The model under review builds one solid part; all positions refer to its coordinate system, in mm. Give positions to 0.01 mm unless a question says otherwise; leave off trailing zeros. Loops run counter-clockwise (first coordinate to the right, second up) from the corner with the lowest first, then second, coordinate; pieces in that order, holes last. Notation, with made-up numbers: (70.5, -3.75) - (120.5, -3.75) arc R8 ccw to (120.5, 0.25) - close; hole circle Ø3 at (33, -9). An arc over 180 degrees is marked (long way). Answer as a JSON object with one key per item and string values.
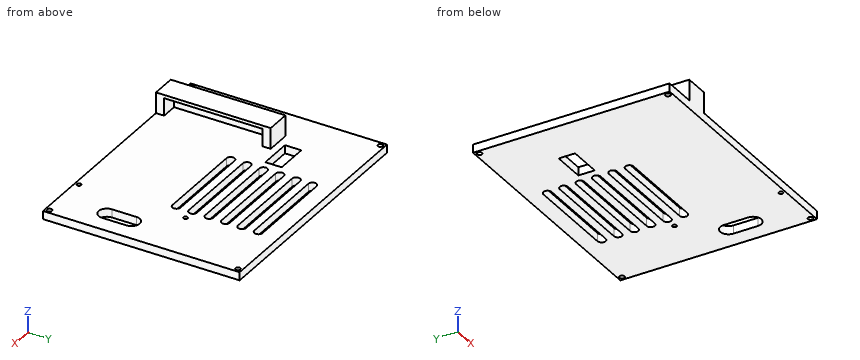
Autodesk Fusion 360 part; units mm, degrees
sketch "スケッチ1" plane through (0, 0, 0) normal (0, 0, 1) x (1, 0, 0)
  line L0 (75, -45) -> (-75, -45)
  line L1 (-75, -45) -> (-75, 75)
  line L2 (-75, 75) -> (75, 75)
  line L3 (75, 75) -> (75, -45)
  line L4 (-115.7726, 0) -> (130, 0)
  dimension "d1" = 150
  dimension "d41" = 75
  dimension "d42" = 45
extrude "押し出し1" add sketch "スケッチ1" along normal blind 5
sketch "スケッチ2" plane through (0, 0, 5) normal (0, 0, 1) x (-1, 0, 0)
  line L0 (-75, -75) -> (75, -75)
  line L1 (75, -75) -> (75, 45)
  line L2 (75, 45) -> (-75, 45)
  line L3 (-75, 45) -> (-75, -75)
  circle A0 centre (72.5, -72.5) radius 1.5
  line L4 (0, -100) -> (0, -20)
  circle A1 centre (-72.5, -72.5) radius 1.5
  line L5 (50, 0) -> (-80, 0)
  circle A2 centre (72.5, 72.5) radius 1.5
  circle A3 centre (-72.5, 72.5) radius 1.5
  dimension "d5" = 3
  dimension "d6" = 2.5
  dimension "d7" = 2.5
extrude "押し出し2" cut sketch "スケッチ2" against normal blind 5 contours A0 | A1 | A2 | A3
sketch "スケッチ3" plane through (0, 0, 5) normal (0, 0, 1) x (-1, 0, 0)
  circle A0 centre (-72.5, -72.5) radius 1.5
  circle A1 centre (72.5, -72.5) radius 1.5
  line L0 (-75, -75) -> (75, -75)
  line L1 (75, -75) -> (75, 45)
  line L2 (75, 45) -> (-75, 45)
  line L3 (-75, 45) -> (-75, -75)
  line L4 (47, -39.5) -> (27, -39.5)
  line L5 (27, -39.5) -> (27, -29.5)
  line L6 (27, -29.5) -> (47, -29.5)
  line L7 (47, -29.5) -> (47, -39.5)
  dimension "d10" = 28
  dimension "d11" = 45.5
  dimension "d12" = 10
  dimension "d13" = 20
extrude "押し出し3" cut sketch "スケッチ3" against normal blind 5 contours L4 L5 L6 L7
sketch "スケッチ4" plane through (0, 0, 5) normal (0, 0, 1) x (-1, 0, 0)
  line L0 (27, -39.5) -> (27, -29.5)
  line L1 (27, -29.5) -> (47, -29.5)
  line L2 (47, -29.5) -> (47, -39.5)
  line L3 (47, -39.5) -> (27, -39.5)
  circle A0 centre (-72.5, -72.5) radius 1.5
  circle A1 centre (72.5, -72.5) radius 1.5
  line L4 (-75, -75) -> (75, -75)
  line L5 (75, -75) -> (75, 45)
  line L6 (75, 45) -> (-75, 45)
  line L7 (-75, 45) -> (-75, -75)
  line L8 (20, -65) -> (-35, -65)
  line L9 (-35, -60) -> (20, -60)
  line L10 (20, -55) -> (-35, -55)
  line L11 (-35, -50) -> (20, -50)
  line L12 (20, -45) -> (-35, -45)
  line L13 (-35, -40) -> (20, -40)
  line L14 (20, -35) -> (-35, -35)
  line L15 (-35, -30) -> (20, -30)
  line L16 (20, -25) -> (-35, -25)
  line L17 (-35, -20) -> (20, -20)
  line L18 (20, -15) -> (-35, -15)
  line L19 (-35, -10) -> (20, -10)
  arc A2 (20, -65) -> (20, -60) centre (20, -62.5) ccw
  arc A3 (20, -55) -> (20, -50) centre (20, -52.5) ccw
  arc A4 (20, -45) -> (20, -40) centre (20, -42.5) ccw
  arc A5 (20, -35) -> (20, -30) centre (20, -32.5) ccw
  arc A6 (20, -25) -> (20, -20) centre (20, -22.5) ccw
  arc A7 (20, -15) -> (20, -10) centre (20, -12.5) ccw
  arc A8 (-35, -10) -> (-35, -15) centre (-35, -12.5) ccw
  arc A9 (-35, -20) -> (-35, -25) centre (-35, -22.5) ccw
  arc A10 (-35, -30) -> (-35, -35) centre (-35, -32.5) ccw
  arc A11 (-35, -40) -> (-35, -45) centre (-35, -42.5) ccw
  arc A12 (-35, -50) -> (-35, -55) centre (-35, -52.5) ccw
  arc A13 (-35, -60) -> (-35, -65) centre (-35, -62.5) ccw
extrude "押し出し4" cut sketch "スケッチ4" against normal blind 5 contours L8 L9 A2 A13 | L10 L11 A3 A12 | L12 L13 A4 A11 | L14 L15 A5 A10 | L16 L17 A6 A9 | L18 L19 A7 A8
sketch "スケッチ5" plane through (0, 0, 5) normal (0, 0, 1) x (-1, 0, 0)
  line L0 (-35, -30) -> (20, -30)
  arc A0 (20, -35) -> (20, -30) centre (20, -32.5) ccw
  line L1 (20, -35) -> (-35, -35)
  arc A1 (-35, -30) -> (-35, -35) centre (-35, -32.5) ccw
  line L2 (-35, -60) -> (20, -60)
  arc A2 (20, -65) -> (20, -60) centre (20, -62.5) ccw
  line L3 (20, -65) -> (-35, -65)
  arc A3 (-35, -60) -> (-35, -65) centre (-35, -62.5) ccw
  line L4 (-35, -50) -> (20, -50)
  arc A4 (20, -55) -> (20, -50) centre (20, -52.5) ccw
  line L5 (20, -55) -> (-35, -55)
  arc A5 (-35, -50) -> (-35, -55) centre (-35, -52.5) ccw
  line L6 (-35, -20) -> (20, -20)
  arc A6 (20, -25) -> (20, -20) centre (20, -22.5) ccw
  line L7 (20, -25) -> (-35, -25)
  arc A7 (-35, -20) -> (-35, -25) centre (-35, -22.5) ccw
  line L8 (-35, -10) -> (20, -10)
  arc A8 (20, -15) -> (20, -10) centre (20, -12.5) ccw
  line L9 (20, -15) -> (-35, -15)
  arc A9 (-35, -10) -> (-35, -15) centre (-35, -12.5) ccw
  line L10 (-35, -40) -> (20, -40)
  arc A10 (20, -45) -> (20, -40) centre (20, -42.5) ccw
  line L11 (20, -45) -> (-35, -45)
  arc A11 (-35, -40) -> (-35, -45) centre (-35, -42.5) ccw
  line L12 (27, -39.5) -> (27, -29.5)
  line L13 (27, -29.5) -> (47, -29.5)
  line L14 (47, -29.5) -> (47, -39.5)
  line L15 (47, -39.5) -> (27, -39.5)
  circle A12 centre (-72.5, -72.5) radius 1.5
  circle A13 centre (72.5, -72.5) radius 1.5
  line L16 (-75, -75) -> (75, -75)
  line L17 (75, -75) -> (75, 45)
  line L18 (75, 45) -> (-75, 45)
  line L19 (-75, 45) -> (-75, -75)
  line L20 (50, -20) -> (40, -20)
  line L21 (40, 40) -> (50, 40)
  line L22 (50, 40) -> (50, -20)
  line L23 (55, -25) -> (40, -25)
  line L24 (40, 45) -> (55, 45)
  line L25 (55, 45) -> (55, -25)
  line L26 (40, -25) -> (40, -20)
  line L27 (40, 40) -> (40, 45)
  circle A14 centre (-52.5, -22.5) radius 1.5
  circle A15 centre (-52.5, 42.5) radius 1.5
  dimension "d18" = 60
  dimension "d20" = 3
  dimension "d21" = 3
  dimension "d22" = 2.5
  dimension "d25" = 2.5
extrude "押し出し5" add sketch "スケッチ5" along normal blind 10.7 contours L18 L20 L21 L22 L23 L24 L25 L26 L27
sketch "スケッチ7" plane through (0, 0, 15.7) normal (0, 0, 1) x (-1, 0, 0)
  line L0 (50, 40) -> (50, -20)
  line L1 (50, -20) -> (40, -20)
  line L2 (40, -20) -> (40, -25)
  line L3 (40, -25) -> (55, -25)
  line L4 (55, -25) -> (55, 45)
  line L5 (55, 45) -> (40, 45)
  line L6 (40, 45) -> (40, 40)
  line L7 (40, 40) -> (50, 40)
  line L8 (55, -25) -> (40, -25)
  line L9 (40, -25) -> (40, 45)
  line L10 (40, 45) -> (55, 45)
  line L11 (55, 45) -> (55, -25)
extrude "押し出し6" add sketch "スケッチ7" along normal blind 2
sketch "スケッチ8" plane through (0, 0, 5) normal (0, 0, 1) x (-1, 0, 0)
  line L0 (50, 40) -> (40, 40)
  line L1 (40, 40) -> (40, 45)
  line L2 (40, 45) -> (-75, 45)
  line L3 (55, 45) -> (55, -25)
  line L4 (55, -25) -> (40, -25)
  line L5 (40, -25) -> (40, -20)
  line L6 (40, -20) -> (50, -20)
  line L7 (50, -20) -> (50, 40)
  line L8 (-35, -30) -> (20, -30)
  arc A0 (20, -35) -> (20, -30) centre (20, -32.5) ccw
  line L9 (20, -35) -> (-35, -35)
  arc A1 (-35, -30) -> (-35, -35) centre (-35, -32.5) ccw
  line L10 (-35, -60) -> (20, -60)
  arc A2 (20, -65) -> (20, -60) centre (20, -62.5) ccw
  line L11 (20, -65) -> (-35, -65)
  arc A3 (-35, -60) -> (-35, -65) centre (-35, -62.5) ccw
  line L12 (-35, -50) -> (20, -50)
  arc A4 (20, -55) -> (20, -50) centre (20, -52.5) ccw
  line L13 (20, -55) -> (-35, -55)
  arc A5 (-35, -50) -> (-35, -55) centre (-35, -52.5) ccw
  line L14 (-35, -20) -> (20, -20)
  arc A6 (20, -25) -> (20, -20) centre (20, -22.5) ccw
  line L15 (20, -25) -> (-35, -25)
  arc A7 (-35, -20) -> (-35, -25) centre (-35, -22.5) ccw
  line L16 (-35, -10) -> (20, -10)
  arc A8 (20, -15) -> (20, -10) centre (20, -12.5) ccw
  line L17 (20, -15) -> (-35, -15)
  arc A9 (-35, -10) -> (-35, -15) centre (-35, -12.5) ccw
  line L18 (-35, -40) -> (20, -40)
  arc A10 (20, -45) -> (20, -40) centre (20, -42.5) ccw
  line L19 (20, -45) -> (-35, -45)
  arc A11 (-35, -40) -> (-35, -45) centre (-35, -42.5) ccw
  line L20 (27, -39.5) -> (27, -29.5)
  line L21 (27, -29.5) -> (47, -29.5)
  line L22 (47, -29.5) -> (47, -39.5)
  line L23 (47, -39.5) -> (27, -39.5)
  circle A12 centre (-72.5, -72.5) radius 1.5
  circle A13 centre (72.5, -72.5) radius 1.5
  line L24 (-75, -75) -> (75, -75)
  line L25 (75, -75) -> (75, 45)
  line L26 (75, 45) -> (55, 45)
  line L27 (-75, 45) -> (-75, -75)
  line L28 (55, -25) -> (-45, -25)
  line L29 (-45, -25) -> (-45, 45)
  line L30 (-45, 45) -> (55, 45)
  line L31 (55, 45) -> (55, -25)
  circle A14 centre (-42.5, -22.5) radius 1.5
  circle A15 centre (-42.5, 42.5) radius 1.5
  dimension "d30" = 3
  dimension "d31" = 2.5
  dimension "d32" = 2.5
  dimension "d33" = 3
  dimension "d34" = 2.5
  dimension "d35" = 2.5
hole "穴1" at (42.5, 22.5, 5) at (42.5, -42.5, 5) direction (0, 0, -1) diameter 2.529 depth 10 tip angle 118
sketch "スケッチ9" plane through (0, 0, 5) normal (0, 0, 1) x (-1, 0, 0)
  circle A0 centre (-42.5, -22.5) radius 1.2645
  circle A1 centre (-42.5, 42.5) radius 1.2645
  line L0 (50, 40) -> (40, 40)
  line L1 (40, 40) -> (40, 45)
  line L2 (40, 45) -> (-75, 45)
  line L3 (55, 45) -> (55, -25)
  line L4 (55, -25) -> (40, -25)
  line L5 (40, -25) -> (40, -20)
  line L6 (40, -20) -> (50, -20)
  line L7 (50, -20) -> (50, 40)
  line L8 (-35, -30) -> (20, -30)
  arc A2 (20, -35) -> (20, -30) centre (20, -32.5) ccw
  line L9 (20, -35) -> (-35, -35)
  arc A3 (-35, -30) -> (-35, -35) centre (-35, -32.5) ccw
  line L10 (-35, -60) -> (20, -60)
  arc A4 (20, -65) -> (20, -60) centre (20, -62.5) ccw
  line L11 (20, -65) -> (-35, -65)
  arc A5 (-35, -60) -> (-35, -65) centre (-35, -62.5) ccw
  line L12 (-35, -50) -> (20, -50)
  arc A6 (20, -55) -> (20, -50) centre (20, -52.5) ccw
  line L13 (20, -55) -> (-35, -55)
  arc A7 (-35, -50) -> (-35, -55) centre (-35, -52.5) ccw
  line L14 (-35, -20) -> (20, -20)
  arc A8 (20, -25) -> (20, -20) centre (20, -22.5) ccw
  line L15 (20, -25) -> (-35, -25)
  arc A9 (-35, -20) -> (-35, -25) centre (-35, -22.5) ccw
  line L16 (-35, -10) -> (20, -10)
  arc A10 (20, -15) -> (20, -10) centre (20, -12.5) ccw
  line L17 (20, -15) -> (-35, -15)
  arc A11 (-35, -10) -> (-35, -15) centre (-35, -12.5) ccw
  line L18 (-35, -40) -> (20, -40)
  arc A12 (20, -45) -> (20, -40) centre (20, -42.5) ccw
  line L19 (20, -45) -> (-35, -45)
  arc A13 (-35, -40) -> (-35, -45) centre (-35, -42.5) ccw
  line L20 (27, -39.5) -> (27, -29.5)
  line L21 (27, -29.5) -> (47, -29.5)
  line L22 (47, -29.5) -> (47, -39.5)
  line L23 (47, -39.5) -> (27, -39.5)
  circle A14 centre (-72.5, -72.5) radius 1.5
  circle A15 centre (72.5, -72.5) radius 1.5
  line L24 (-75, -75) -> (75, -75)
  line L25 (75, -75) -> (75, 45)
  line L26 (75, 45) -> (55, 45)
  line L27 (-75, 45) -> (-75, -75)
  line L28 (-65, 0) -> (-65, 15)
  line L29 (-55, 15) -> (-55, 0)
  arc A16 (-65, 0) -> (-55, 0) centre (-60, 0) ccw
  arc A17 (-55, 15) -> (-65, 15) centre (-60, 15) ccw
extrude "押し出し7" cut sketch "スケッチ9" against normal blind 5 contours L28 L29 A16 A17
sketch "スケッチ10" plane through (0, 0, 5) normal (0, 0, 1) x (-1, 0, 0)
  line L0 (-55, 15) -> (-55, 0)
  arc A0 (-65, 0) -> (-55, 0) centre (-60, 0) ccw
  line L1 (-65, 0) -> (-65, 15)
  arc A1 (-55, 15) -> (-65, 15) centre (-60, 15) ccw
  circle A2 centre (-42.5, -22.5) radius 1.2645
  circle A3 centre (-42.5, 42.5) radius 1.2645
  line L2 (55, 45) -> (55, -25)
  line L3 (55, -25) -> (40, -25)
  line L4 (40, -25) -> (40, -20)
  line L5 (40, -20) -> (50, -20)
  line L6 (50, -20) -> (50, 40)
  line L7 (50, 40) -> (40, 40)
  line L8 (40, 40) -> (40, 45)
  line L9 (40, 45) -> (-75, 45)
  line L10 (-75, 45) -> (-75, -75)
  line L11 (-75, -75) -> (75, -75)
  line L12 (75, -75) -> (75, 45)
  line L13 (75, 45) -> (55, 45)
  circle A4 centre (72.5, -72.5) radius 1.5
  circle A5 centre (-72.5, -72.5) radius 1.5
  line L14 (27, -39.5) -> (27, -29.5)
  line L15 (27, -29.5) -> (47, -29.5)
  line L16 (47, -29.5) -> (47, -39.5)
  line L17 (47, -39.5) -> (27, -39.5)
  line L18 (-35, -40) -> (20, -40)
  arc A6 (20, -45) -> (20, -40) centre (20, -42.5) ccw
  line L19 (20, -45) -> (-35, -45)
  arc A7 (-35, -40) -> (-35, -45) centre (-35, -42.5) ccw
  line L20 (-35, -10) -> (20, -10)
  arc A8 (20, -15) -> (20, -10) centre (20, -12.5) ccw
  line L21 (20, -15) -> (-35, -15)
  arc A9 (-35, -10) -> (-35, -15) centre (-35, -12.5) ccw
  line L22 (-35, -20) -> (20, -20)
  arc A10 (20, -25) -> (20, -20) centre (20, -22.5) ccw
  line L23 (20, -25) -> (-35, -25)
  arc A11 (-35, -20) -> (-35, -25) centre (-35, -22.5) ccw
  line L24 (-35, -50) -> (20, -50)
  arc A12 (20, -55) -> (20, -50) centre (20, -52.5) ccw
  line L25 (20, -55) -> (-35, -55)
  arc A13 (-35, -50) -> (-35, -55) centre (-35, -52.5) ccw
  line L26 (-35, -60) -> (20, -60)
  arc A14 (20, -65) -> (20, -60) centre (20, -62.5) ccw
  line L27 (20, -65) -> (-35, -65)
  arc A15 (-35, -60) -> (-35, -65) centre (-35, -62.5) ccw
  line L28 (-35, -30) -> (20, -30)
  arc A16 (20, -35) -> (20, -30) centre (20, -32.5) ccw
  line L29 (20, -35) -> (-35, -35)
  arc A17 (-35, -30) -> (-35, -35) centre (-35, -32.5) ccw
  circle A18 centre (72.5, 42.5) radius 1.5
  circle A19 centre (-72.5, 42.5) radius 1.5
  dimension "d43" = 3
  dimension "d44" = 2.5
  dimension "d45" = 2.5
  dimension "d46" = 3
  dimension "d47" = 2.5
  dimension "d48" = 2.5
extrude "押し出し8" cut sketch "スケッチ10" against normal blind 5 contours A18 | A19
equation "d11 = 35 mm + 10.50 mm"
equation "d42 = 75 mm - 30 mm"
Q1. To check wall thickness, follow probe 1 along Y at (x, z) = (-72.5, 2.2); probe 2 along X at (y, z) = (-42.5, 3.7); probe 3 along X at (y, z) = (22.5, 3.85). State the ranges of each line that lie inside material, in increasing order. Write a range as [from, to].
Results:
{"probe 1": "y = [-45, -44], [-41, 71], [74, 75]", "probe 2": "x = [-75, -74], [-71, 41.24], [43.76, 71], [74, 75]", "probe 3": "x = [-75, -22.5], [37.5, 41.24], [43.76, 75]"}
Q2. Consider section C-C, the plane x = -12.5. State the section outline as (y, z) points.
Results:
{"outline": "(-45, 0) - (10, 0) - (10, 5) - (-45, 5) - close; (15, 0) - (20, 0) - (20, 5) - (15, 5) - close; (25, 0) - (30, 0) - (30, 5) - (25, 5) - close; (35, 0) - (40, 0) - (40, 5) - (35, 5) - close; (45, 0) - (50, 0) - (50, 5) - (45, 5) - close; (55, 0) - (60, 0) - (60, 5) - (55, 5) - close; (65, 0) - (75, 0) - (75, 5) - (65, 5) - close"}
Q3. Consider section A-A, the plane y = 62.5. State the section outline as (x, z) points.
Results:
{"outline": "(-75, 0) - (-22.5, 0) - (-22.5, 5) - (-75, 5) - close; (37.5, 0) - (75, 0) - (75, 5) - (37.5, 5) - close"}
Q4. Consider section D-D, the plane z = 13.75. State the section outline as (x, y) points.
Results:
{"outline": "(-55, -45) - (-40, -45) - (-40, -40) - (-50, -40) - (-50, 20) - (-40, 20) - (-40, 25) - (-55, 25) - close"}
Q5. Consider section B-B, the plane x = 60. State the section outline as (y, z) points.
Results:
{"outline": "(-45, 0) - (-20, 0) - (-20, 5) - (-45, 5) - close; (5, 0) - (75, 0) - (75, 5) - (5, 5) - close"}
Q6. Clearance check with flat-ended pins moving along their axes: pin 1 Ø3 at (x, z) = (-44, 9.5) entering from +Y; pin 2 Ø4 at (y, z) = (-19, 8) entering from -X; pin 3 Ø12 at (x, y) = (-29.5, -16.5) entering from +Z. State where each tip first meets the part, or that it passes through.
Results:
{"pin 1": "stops at y = 25", "pin 2": "stops at x = -55", "pin 3": "stops at z = 5"}
